Here's how the part is built. I have some questions about the finished solid (model axes, mm). Give positions to 0.01 mm unless a question says otherwise; leave off trailing zeros. Loops run counter-clockwise (first coordinate to the right, second up) from the corner with the lowest first, then second, coordinate; pieces in that order, holes last. Notation, with made-up numbers: (-32, 56) - (10, 56) arc R12 ccw to (10, 75) - close; hole circle Ø8 at (9, 1). An arc over 180 degrees is marked (long way). One line per item, written item: value. Start each with the question number.
```python
from build123d import *

# Parameters (mm, degrees)
ESBO_O1_R                = 2.5
RESSALTO_EXTRUS_O1_DEPTH = 160
ESBO_O2_R                = 1.5
CORTE_EXTRUS_O1_DEPTH    = 16.714243329
ESBO_O3_R                = 1.5
CORTE_EXTRUS_O2_DEPTH    = 16.714243329


with BuildPart() as part:
    # Esboço1 → Ressalto-extrusão1 (new body)
    with BuildSketch(Plane.XY):
        Polygon((5.897209639, -4.357321633), (6.722156046, 2.928472542), (0.824946407, 7.285794175), (-5.897209639, 4.357321633), (-6.722156046, -2.928472542), (-0.824946407, -7.285794175), align=None)
        Circle(ESBO_O1_R, mode=Mode.SUBTRACT)
    extrude(amount=RESSALTO_EXTRUS_O1_DEPTH)

    # Esboço2 → Corte-extrusão1 (cut, through all)
    with BuildSketch(Plane(origin=(-2.536131616, 5.821557904, 0), x_dir=(0.916780772, 0.399390806, 0), z_dir=(-0.399390806, 0.916780772, 0))):
        with Locations((0, -57)):
            Circle(ESBO_O2_R)
    extrude(amount=-CORTE_EXTRUS_O1_DEPTH, mode=Mode.SUBTRACT)

    # Esboço3 → Corte-extrusão2 (cut, through all)
    with BuildSketch(Plane(origin=(-2.536131616, 5.821557904, 0), x_dir=(0.916780772, 0.399390806, 0), z_dir=(-0.399390806, 0.916780772, 0))):
        with Locations((0, -128.44)):
            Circle(ESBO_O3_R)
    extrude(amount=-CORTE_EXTRUS_O2_DEPTH, mode=Mode.SUBTRACT)


solid = part.part
```
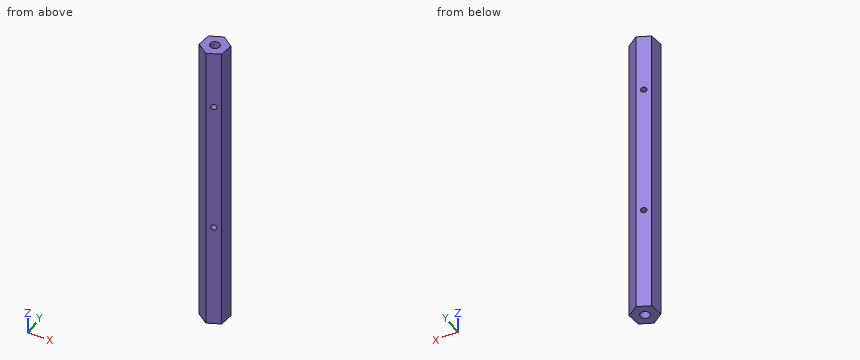
(1) If we section it at A-A on z = 64.5: List the corners of the cut face in (x, y) for me.
(2) Please list where these lines run through material, in increasing order: probe 1 along Z at (x, y) = (-2, 4.75); probe 2 along Z at (x, y) = (-3, 5); probe 3 along X at (y, z) = (2.25, 132). Write a range as from..to.
(3) Will these pins go through, and if not, where does the flat tip stop? pin 1 (4.5 mm diameter, centred on x = 0, y = 0, fed in from +Z); pin 2 (3 mm diameter, centred on x = 3, z = 22.5, fed in from -Y); pin 3 (3 mm diameter, centred on x = -3.5, z = 45.5, fed in from +Y); pin 4 (5 mm diameter, centred on y = -1, z = 40, fed in from +X).
Found:
1. outline: (-6.72, -2.93) - (-0.82, -7.29) - (5.9, -4.36) - (6.72, 2.93) - (0.82, 7.29) - (-5.9, 4.36) - close; hole circle Ø5 at (0, 0)
2. probe 1: 0..55.5, 58.5..126.94, 129.94..160
2. probe 2: 0..55.7, 58.3..127.14, 129.74..160
2. probe 3: -6.14..-1.09, 1.09..6.65
3. pin 1: through
3. pin 2: y = -6.27
3. pin 3: y = 6.06
3. pin 4: x = 6.56
